Input: part model. Units: mm. Frame: model coordinates. A direction names the side the tool comes from. Round coordinates to 2 decimals unless told otherwise and drop trailing zeros. Order: outer loops, then holes, each group sorted by start corner. A loop starts at its lowest first (then second) coordinate and runs counter-clockwise, first axis right, second up.
Item 1: Reachability of faces 1 (the flat face through (0, 34, 5.25)), 2 (the flat face through (-17.5, 34, 4)) from +Z, -Z, +X, -X, +Y, -Y: full face, straight path, thin tool, end or side. Return the list, or none.
Item 2: Cut plane A-A on y = -48.26. Output: boundary loops of the cut face in (x, z) (3 decimals), then the cut area to 3 significant figures.
Item 3: Cut plane C-C on y = -13. Output: boundary loops of the cut face in (x, z) (3 decimals).
Item 4: Cut plane B-B on x = -10. Output: boundary loops of the cut face in (y, z), then the cut area to 3 significant figures.
Item 5: Cut plane D-D on x = 0. Give the number of separate pieces and of enclosed holes in the cut face, then the cut area to 3 significant figures.
Item 6: Mould query, pull axis X, two halves, no side actions, for faces 3 (the flat face through (0, 36, 4)), 4 (the flat face through (0, -57.15, 4)), 5 (the cylindrical face through (-11.8, -12.92, 1.49)), 6 (the flat face through (34.925, -1, 4)). Classes: released by +X, released by -X, zero draft, split by the parting line, or undercut.
Item 7: First-contact query: pin 1 (3 mm diameter, centred on x = -8, z = 1, fed in from +Y); pin 2 (7.5 mm diameter, centred on x = 0, y = -48.26, fed in from -Z); pin 3 (5 mm diameter, centred on x = 19, y = -6.5, fed in from +Z). Flat tips, straight axial feed; report the tip coordinate or a pass-through.
Item 8: Line query: L1, parallel to Y at x = 7, z = 3.75; L2, parallel to Y at x = 23, z = 4.45; L3, parallel to X at y = -13, z = 1.8. Output: solid intervals per line, ascending.
```python
from build123d import *

# Parameters (mm, degrees)
SKETCH_W      = 69.85
SKETCH_H      = 114.3
SKETCH_R      = 2.3
SKETCH_R_2    = 6.5
SKETCH_R_3    = 1.8
PAD_DEPTH     = 5.25
FILLET_R      = 1
CHAMFER_SIZE  = 1.5
FILLET001_R   = 1
FILLET002_R   = 3
SKETCH001_W   = 65.85
SKETCH001_H   = 110.3
SKETCH001_W_2 = 35
SKETCH001_H_2 = 4
POCKET_DEPTH  = 3.25
FILLET003_R   = 2


with BuildPart() as part:
    # Sketch → Pad (new body)
    with BuildSketch(Plane.XY):
        Rectangle(SKETCH_W, SKETCH_H)
        with Locations((0, 48.26)):
            Circle(SKETCH_R, mode=Mode.SUBTRACT)
        with Locations((0, -48.26)):
            Circle(SKETCH_R, mode=Mode.SUBTRACT)
        with Locations((0, 19)):
            Circle(SKETCH_R_2, mode=Mode.SUBTRACT)
        with Locations((-10, -13)):
            Circle(SKETCH_R_3, mode=Mode.SUBTRACT)
        with Locations((10, -13)):
            Circle(SKETCH_R_3, mode=Mode.SUBTRACT)
    extrude(amount=PAD_DEPTH)

    # Fillet
    fillet_edges = [part.edges().sort_by_distance(p)[0] for p in [
        (-6.5, 19, 0),
    ]]
    fillet(fillet_edges, radius=FILLET_R)

    # Chamfer
    chamfer_edges = [part.edges().sort_by_distance(p)[0] for p in [
        (-2.3, 48.26, 0),
        (-2.3, -48.26, 0),
    ]]
    chamfer(chamfer_edges, length=CHAMFER_SIZE)

    # Fillet001
    fillet001_edges = [part.edges().sort_by_distance(p)[0] for p in [
        (-11.8, -13, 0),
        (8.2, -13, 0),
    ]]
    fillet(fillet001_edges, radius=FILLET001_R)

    # Fillet002
    fillet002_edges = [part.edges().sort_by_distance(p)[0] for p in [
        (0, 57.15, 0),
        (-34.925, 0, 0),
        (34.925, 0, 0),
        (0, -57.15, 0),
    ]]
    fillet(fillet002_edges, radius=FILLET002_R)

    # Sketch001 (on Face20 of Fillet002) → Pocket (cut)
    with BuildSketch(Plane.XY.offset(5.25)):
        Rectangle(SKETCH001_W, SKETCH001_H)
        with Locations((0, 34)):
            Rectangle(SKETCH001_W_2, SKETCH001_H_2, mode=Mode.SUBTRACT)
        with Locations((0, -34)):
            Rectangle(SKETCH001_W_2, SKETCH001_H_2, mode=Mode.SUBTRACT)
    extrude(amount=-POCKET_DEPTH, mode=Mode.SUBTRACT)

    # Fillet003
    fillet003_edges = [part.edges().sort_by_distance(p)[0] for p in [
        (-32.925, 0, 2),
        (0, 55.15, 2),
        (32.925, 0, 2),
        (0, -55.15, 2),
    ]]
    fillet(fillet003_edges, radius=FILLET003_R)


solid = part.part
```
From the geometry:
1. face 1: +Z, +X, -X, +Y, -Y
1. face 2: +Z
2. outline: (-34.925, 3) arc R3 ccw to (-31.925, 0) - (-3.8, 0) - (-2.3, 1.5) - (-2.3, 2) - (-30.925, 2) arc R2 cw to (-32.925, 4) - (-32.925, 5.25) - (-34.925, 5.25) - close; (2.3, 1.5) - (3.8, 0) - (31.925, 0) arc R3 ccw to (34.925, 3) - (34.925, 5.25) - (32.925, 5.25) - (32.925, 4) arc R2 cw to (30.925, 2) - (2.3, 2) - close
2. area: 139 mm2
3. outline: (-34.925, 3) arc R3 ccw to (-31.925, 0) - (-12.8, 0) arc R1 ccw to (-11.8, 1) - (-11.8, 2) - (-30.925, 2) arc R2 cw to (-32.925, 4) - (-32.925, 5.25) - (-34.925, 5.25) - close; (-8.2, 1) arc R1 ccw to (-7.2, 0) - (7.2, 0) arc R1 ccw to (8.2, 1) - (8.2, 2) - (-8.2, 2) - close; (11.8, 1) arc R1 ccw to (12.8, 0) - (31.925, 0) arc R3 ccw to (34.925, 3) - (34.925, 5.25) - (32.925, 5.25) - (32.925, 4) arc R2 cw to (30.925, 2) - (11.8, 2) - close
4. outline: (-57.15, 3) arc R3 ccw to (-54.15, 0) - (-15.8, 0) arc R1 ccw to (-14.8, 1) - (-14.8, 2) - (-32, 2) - (-32, 5.25) - (-36, 5.25) - (-36, 2) - (-53.15, 2) arc R2 cw to (-55.15, 4) - (-55.15, 5.25) - (-57.15, 5.25) - close; (-11.2, 1) arc R1 ccw to (-10.2, 0) - (54.15, 0) arc R3 ccw to (57.15, 3) - (57.15, 5.25) - (55.15, 5.25) - (55.15, 4) arc R2 cw to (53.15, 2) - (36, 2) - (36, 5.25) - (32, 5.25) - (32, 2) - (-11.2, 2) - close
4. area: 258 mm2
5. separate pieces: 4
5. enclosed holes: 0
5. area: 216 mm2
6. face 3: undercut
6. face 4: zero draft
6. face 5: undercut
6. face 6: released by +X
7. pin 1: stops at y = 57.11
7. pin 2: stops at z = 0.05
7. pin 3: stops at z = 2
8. L1: y = -57.15 to -55.13, -36 to -32, 32 to 36, 55.13 to 57.15
8. L2: y = -57.15 to -55.15, 55.15 to 57.15
8. L3: x = -34.67 to -11.8, -8.2 to 8.2, 11.8 to 34.67
